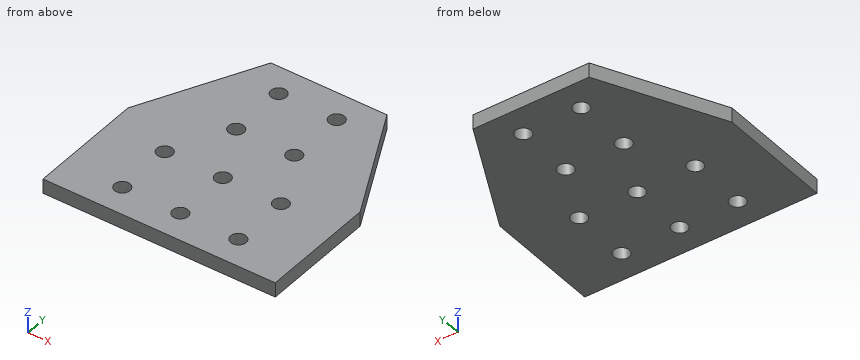
```python
from build123d import *

# Parameters (mm, degrees)
F0_R     = 3.3782
F1_DEPTH = 6.35


with BuildPart() as f1:
    # F0 (on Top) → F1 (new body)
    with BuildSketch(Plane.XY):
        Polygon((76.2, 0), (25.4, 0), (0, -50.8), (0, -101.6), (101.6, -101.6), (101.6, -50.8), align=None)
        with Locations((25.4, -88.9)):
            Circle(F0_R, mode=Mode.SUBTRACT)
        with Locations((50.8, -88.9)):
            Circle(F0_R, mode=Mode.SUBTRACT)
        with Locations((25.4, -63.5)):
            Circle(F0_R, mode=Mode.SUBTRACT)
        with Locations((50.8, -63.5)):
            Circle(F0_R, mode=Mode.SUBTRACT)
        with Locations((76.2, -88.9)):
            Circle(F0_R, mode=Mode.SUBTRACT)
        with Locations((76.2, -63.5)):
            Circle(F0_R, mode=Mode.SUBTRACT)
        with Locations((38.1, -38.1)):
            Circle(F0_R, mode=Mode.SUBTRACT)
        with Locations((38.1, -12.7)):
            Circle(F0_R, mode=Mode.SUBTRACT)
        with Locations((63.5, -38.1)):
            Circle(F0_R, mode=Mode.SUBTRACT)
        with Locations((63.5, -12.7)):
            Circle(F0_R, mode=Mode.SUBTRACT)
    extrude(amount=F1_DEPTH)


solid = f1.part
```
Here's how the part is built. I have some questions about the finished solid (model axes, mm). Round coordinates to 2 decimals unless told otherwise and drop trailing zeros. Order: outer loops, then holes, each group sorted by start corner. A loop starts at its lowest first (then second) coordinate and runs counter-clockwise, first axis right, second up. Notation, with made-up numbers: (-35.5, 2) -> (0.5, 2) arc R27 ccw to (0.5, 31) -> close; hole circle Ø5 at (33, 60.5). An arc over 180 degrees is marked (long way). Use a Markdown table: item, result. Add a question column.
(1) Suppose I cut it at B-B, the plane x = 38.1. Please give me the cut outline in (y, z), and give its area (3 significant figures).
(2) For pin 1 Ø6 at (x, y) = (52, -15.5) entering from -Z; pin 2 Ø3 at (x, z) = (91, 4.5) entering from +Y; pin 3 Ø1 at (x, z) = (23.5, 4.5) entering from +Y, each with a flat end and sliding along its axis, tell me the tip position at first contact or that it passes through.
(3) Suppose I cut it at D-D, the plane y = -12.7. Please give me the cut outline in (x, z), and give its area (3 significant figures).
(4) Suppose I cut it at C-C, the plane z = 1. Count the separate pieces of the cut face and the enclosed holes in it, and give its area (3 significant figures).
(5) I need wall thicknesses on line 1 along Y through (x, z) = (38.1, 2.25); line 2 along Y through (x, z) = (50.8, 4.25); line 3 along X through (y, z) = (-61, 3). Which ranges of each line are inside material? Lowest first, please.
(6) Suppose I cut it at A-A, the plane y = -63.5. Please give me the cut outline in (x, z).
Verdict:
| question | item | result |
|---|---|---|
| 1 | outline | (-101.6, 0) -> (-41.48, 0) -> (-41.48, 6.35) -> (-101.6, 6.35) -> close; (-34.72, 0) -> (-16.08, 0) -> (-16.08, 6.35) -> (-34.72, 6.35) -> close; (-9.32, 0) -> (0, 0) -> (0, 6.35) -> (-9.32, 6.35) -> close |
| 1 | area | 559 mm2 |
| 2 | pin 1 | z = 0 |
| 2 | pin 2 | y = -26.6 |
| 2 | pin 3 | y = -2.8 |
| 3 | outline | (19.05, 0) -> (34.72, 0) -> (34.72, 6.35) -> (19.05, 6.35) -> close; (41.48, 0) -> (60.12, 0) -> (60.12, 6.35) -> (41.48, 6.35) -> close; (66.88, 0) -> (82.55, 0) -> (82.55, 6.35) -> (66.88, 6.35) -> close |
| 3 | area | 317 mm2 |
| 4 | separate pieces | 1 |
| 4 | enclosed holes | 10 |
| 4 | area | 8,670 mm2 |
| 5 | line 1 | -101.6 to -41.48, -34.72 to -16.08, -9.32 to 0 |
| 5 | line 2 | -101.6 to -92.28, -85.52 to -66.88, -60.12 to 0 |
| 5 | line 3 | 0 to 23.13, 27.67 to 48.53, 53.07 to 73.93, 78.47 to 101.6 |
| 6 | outline | (0, 0) -> (22.02, 0) -> (22.02, 6.35) -> (0, 6.35) -> close; (28.78, 0) -> (47.42, 0) -> (47.42, 6.35) -> (28.78, 6.35) -> close; (54.18, 0) -> (72.82, 0) -> (72.82, 6.35) -> (54.18, 6.35) -> close; (79.58, 0) -> (101.6, 0) -> (101.6, 6.35) -> (79.58, 6.35) -> close |
